Input: part model. Units: mm. Frame: model coordinates. Face numbers are marked on the shaded views. A direction names the side the tool comes from. Coordinates: 2 decimals unless noted, no trailing zeros. Loops run counter-clockwise (first coordinate to the right, second up) from the corner with the lowest first, then second, coordinate; pieces in that order, holes last.
(1) Section D-D, the plane x = -30. Return loops of the section in (y, z), then the cut area to 3 significant figures.
(2) Section B-B, the plane y = 9.75. Return loops of the section in (x, z), then the cut area to 3 significant figures.
(3) Line query: L1, parallel to X at y = 9.5, z = -20; L2, parallel to Z at x = 7.5, y = -1; L3, parallel to Z at x = 10, y = -6.25. Output: solid intervals per line, ascending.
(4) Section C-C, the plane x = 25.5. Return loops of the section in (y, z).
(5) Section A-A, the plane x = 14. Return loops of the section in (y, z).
(6) Contact query for flat-ended pins moving along their axis: P1, Ø4, axis at y = -1.5, z = 4.5, coming from the +X side; P2, Ø5, axis at x = 26, y = 2.5, coming from the +Z side; P3, Ø1, axis at y = -0.5, z = 38.5, coming from the +X side. Output: stop coordinate, or through.
(7) Set-up query: the marked faces 4, 5, 6 and 7. Return all of +Z, -Z, +X, -X, +Y, -Y with unobstructed straight access to the full face (end or side cutting, diameter ignored); none if empty.
(8) Mould query, pull axis X, two halves, no side actions, for the marked faces 1, 2 and 3. Classes: released by +X, released by -X, zero draft, split by the parting line, or undercut.
```python
from build123d import *

# Parameters (mm, degrees)
F1_DEPTH = 12.5
F2_DEPTH = 5


with BuildPart() as f1:
    # F0 (on Front) → F1 (new body, symmetric)
    with BuildSketch(Plane.XZ):
        with BuildLine():
            Line((-47.340788, -33.865508), (47.340788, -33.865508))
            Line((47.340788, -33.865508), (47.340788, 6.859001))
            ThreePointArc((47.340788, 6.859001), (28.244304, 14.769024), (20.334281, 33.865508))
            Line((20.334281, 33.865508), (0, 33.865508))
            Line((0, 33.865508), (-47.340788, 33.865508))
            Line((-47.340788, 33.865508), (-47.340788, -33.865508))
        make_face()
    extrude(amount=F1_DEPTH, both=True)

    # F0 (on Front) → F2 (join, symmetric)
    with BuildSketch(Plane.XZ):
        with BuildLine():
            ThreePointArc((50.061827, 60.734585), (-3.651514, 65.469078), (-47.340788, 33.865508))
            Line((-47.340788, 33.865508), (0, 33.865508))
            ThreePointArc((0, 33.865508), (7.223757, 54.839315), (29.392478, 54.044942))
            ThreePointArc((29.392478, 54.044942), (39.024823, 59.55979), (50.061827, 60.734585))
        make_face()
    extrude(amount=F2_DEPTH, both=True)


solid = f1.part
```
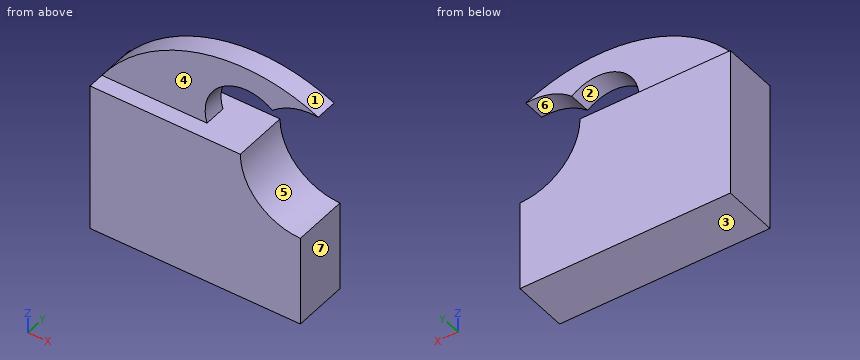
Report:
1. outline: (-12.5, -33.87) - (12.5, -33.87) - (12.5, 33.87) - (5, 33.87) - (5, 52.38) - (-5, 52.38) - (-5, 33.87) - (-12.5, 33.87) - close
1. area: 1,880 mm2
2. outline: (-47.34, -33.87) - (47.34, -33.87) - (47.34, 6.86) arc R27.01 cw to (20.33, 33.87) - (-47.34, 33.87) - close
2. area: 5,840 mm2
3. L1: x = -47.34 to 47.34
3. L2: z = -33.87 to 33.87, 55.03 to 67.68
3. L3: z = -33.87 to 33.87
4. outline: (-12.5, -33.87) - (12.5, -33.87) - (12.5, 17.98) - (-12.5, 17.98) - close; (-5, 56.43) - (5, 56.43) - (5, 67.76) - (-5, 67.76) - close
5. outline: (-12.5, -33.87) - (12.5, -33.87) - (12.5, 33.87) - (-12.5, 33.87) - close; (-5, 57.73) - (5, 57.73) - (5, 68.19) - (-5, 68.19) - close
6. P1: stops at x = 47.34
6. P2: stops at z = 67.96
6. P3: stops at x = -0.81
7. face 4: +Z, +X, -X, -Y
7. face 5: +X, +Y, -Y
7. face 6: +Y, -Y
7. face 7: -Z, +X, +Y, -Y
8. face 1: split by the parting line
8. face 2: undercut
8. face 3: zero draft
